Autodesk Inventor part; units mm, degrees
ref_plane "YZ Plane" through (0, 0, 0) normal (1, 0, 0) x (0, 1, 0)
ref_plane "XZ Plane" through (0, 0, 0) normal (0, 1, 0) x (-1, 0, 0)
ref_plane "XY Plane" through (0, 0, 0) normal (0, 0, 1) x (1, 0, 0)
sketch "Sketch1" plane through (0, 0, 0) normal (0, 0, 1) x (1, 0, 0)
  line L0 (-192.5, 35) -> (192.5, 35)
  line L1 (192.5, 35) -> (192.5, -55)
  line L2 (192.5, -55) -> (-192.5, -55)
  line L3 (-192.5, -55) -> (-192.5, 35)
  point P0 (0, 0)
  dimension "d0" = 385
  dimension "d1" = 192.5
  dimension "d2" = 90
  dimension "d3" = 55
extrude "Extrusion1" add sketch "Sketch1" along normal blind 7
sketch "Sketch2" plane through (0, 0, 0) normal (0, 0, -1) x (-1, 0, 0)
  line L0 (192.5, 35) -> (-192.5, 35)
  line L1 (-192.5, 35) -> (-192.5, -55)
  line L2 (-192.5, -55) -> (192.5, -55)
  line L3 (17.417, 16.6256) -> (17.417, -16.6484)
  line L4 (-192.5, 16.6256) -> (-192.5, -16.6484)
  line L5 (17.417, 35) -> (17.417, -55)
  line L6 (4.717, 16.6256) -> (4.717, -16.6484)
  line L7 (-171.164, 18.034) -> (-179.8, 18.034)
  line L8 (-179.8, 16.6256) -> (-179.8, -16.6484)
  line L9 (-179.8, 35) -> (-179.8, -55)
  line L10 (4.717, 35) -> (4.717, -55)
  point P0 (0, 0)
extrude "Extrusion2" add sketch "Sketch2" along normal blind 4.7408 contours L5 L3 L2 L10 L6 L0 | L9 L8 L2 L1 L0
sketch "Sketch3" plane through (0, 0, 0) normal (0, 0, -1) x (-1, 0, 0)
  line L0 (17.417, 35) -> (17.417, -55)
  line L1 (17.417, -55) -> (192.5, -55)
  line L2 (63.2414, 16.4628) -> (60.0979, -19.4679)
  line L3 (17.417, 35) -> (67.417, 35)
  line L4 (67.417, 35) -> (67.417, -55)
  line L5 (67.417, -55) -> (17.417, -55)
  line L6 (17.417, -55) -> (17.417, 35)
  line L7 (76.6696, -19.4) -> (76.6696, 30.6)
  line L8 (17.417, 35) -> (76.6696, 35)
  line L9 (76.6696, -55) -> (17.417, -55)
  line L10 (17.417, -55) -> (17.417, 35)
  circle A0 centre (83.6696, -4.5) radius 1.5
  circle A1 centre (83.6696, 10.5) radius 2
  line L11 (87.4689, -18.5) -> (87.4689, -24.5)
  line L12 (88.6696, -24.5) -> (87.4689, -24.5)
  line L13 (88.6696, 15.5) -> (88.6696, -24.5)
  line L14 (78.6696, 15.5) -> (88.6696, 15.5)
  line L15 (78.6696, -15.5) -> (78.6696, 15.5)
  line L16 (78.6696, -15.5) -> (84.4689, -15.5)
  arc A2 (87.4689, -18.5) -> (84.4689, -15.5) centre (84.4689, -18.5) ccw
  line L17 (67.417, 35) -> (78.6696, 35)
  line L18 (78.6696, 35) -> (78.6696, -55)
  line L19 (78.6696, -55) -> (67.417, -55)
  line L20 (67.417, -55) -> (67.417, 35)
  point P0 (0, 0)
  dimension "d8" = 50
  dimension "d11" = 0
extrude "Extrusion3" add sketch "Sketch3" along normal blind 7.3198 contours L3 L4 L1 L0 | L8 L17 L18 L15 L1 L4
sketch "Sketch6" plane through (-192.5, -55, 7) normal (-1, 0, 0) x (0, 0, 1)
  line L0 (-23, 0) -> (-23, 65)
  circle A0 centre (-28, 23.1) radius 1.2295
  circle A1 centre (-28, 53.1) radius 1.2295
  point P0 (-7, 55)
hole "Hole1" at (-192.5, -31.9, -21) at (-192.5, -1.9, -21) direction (1, 0, 0) diameter 3 end through all counterbore diameter 5.75 counterbore depth 3
sketch "Sketch8" plane through (0, 0, 7) normal (0, 0, 1) x (1, 0, 0)
  circle A0 centre (-57.2416, -1.1152) radius 2.0828
  circle A1 centre (-33.7068, 0.9439) radius 2.0828
  point P0 (0, 0)
hole "Hole3" [suppressed]
sketch "Sketch9" plane through (0, 0, -4.7408) normal (0, 0, -1) x (-1, 0, 0)
  circle A0 centre (11.067, -7.6314) radius 2.1844
  circle A1 centre (11.067, 7.6086) radius 2.1844
  circle A2 centre (-186.15, -7.6314) radius 2.1844
  circle A3 centre (-186.15, 7.6086) radius 2.1844
  point P0 (0, 0)
hole "Hole4" at (-11.067, -7.6314, -4.7408) at (-11.067, 7.6086, -4.7408) at (186.15, -7.6314, -4.7408) at (186.15, 7.6086, -4.7408) direction (0, 0, 1) diameter 3.302 depth 8 tip angle 118
sketch "Sketch10" plane through (0, 0, 0) normal (0, 0, -1) x (-1, 0, 0)
  line L0 (192.5, 35) -> (78.6696, 35)
  line L1 (178.6696, 15.5) -> (178.6696, -24.5)
  line L2 (178.6696, 35) -> (192.5, 35)
  line L3 (192.5, 35) -> (192.5, -55)
  line L4 (192.5, -55) -> (178.6696, -55)
  line L5 (178.6696, -55) -> (178.6696, 35)
  point P0 (0, 0)
extrude "Extrusion6" cut sketch "Sketch10" against normal blind 10
sketch "Sketch11" plane through (0, 0, 0) normal (0, 0, -1) x (-1, 0, 0)
  line L0 (178.6696, -55) -> (178.6696, 35)
  line L1 (178.6696, 35) -> (78.6696, 35)
  line L2 (78.6696, 35) -> (78.6696, -55)
  line L3 (78.6696, -55) -> (178.6696, -55)
  point P0 (0, 0)
extrude "Extrusion7" add sketch "Sketch11" along normal blind 7.3198
sketch "Sketch12" plane through (0, 0, -7.3198) normal (0, 0, -1) x (-1, 0, 0)
  circle A0 centre (173.6696, 10.5) radius 2
  line L0 (78.6696, 15.5) -> (178.6696, 15.5)
  line L1 (178.6696, 15.5) -> (178.6696, -24.5)
  line L2 (178.6696, -24.5) -> (78.6696, -24.5)
  line L3 (78.6696, -24.5) -> (78.6696, 15.5)
  circle A1 centre (173.6696, -44.5) radius 2.0242
  circle A2 centre (58.6696, 10.5) radius 2.0032
  circle A3 centre (58.6696, -44.5) radius 2.0032
  point P0 (0, 0)
  dimension "d126" = 55
  dimension "d127" = 115
hole "Hole5" at (-173.6696, 10.5, -7.3198) direction (0, 0, 1) diameter 2.459 depth 8.8 tip angle 118
sketch "Sketch13" plane through (0, 0, -7.3198) normal (0, 0, -1) x (-1, 0, 0)
  line L0 (171.6696, -6) -> (175.6696, -6)
  arc A0 (175.6696, -6) -> (175.6696, -3) centre (175.6696, -4.5) ccw
  line L1 (175.6696, -3) -> (171.6696, -3)
  arc A1 (171.6696, -3) -> (171.6696, -6) centre (171.6696, -4.5) ccw
  circle A2 centre (83.6696, -4.5) radius 1.5
  circle A3 centre (173.6696, 10.5) radius 2
  circle A4 centre (173.6696, -19.5) radius 2
  circle A5 centre (83.6696, 10.5) radius 2
  circle A6 centre (83.6696, -19.5) radius 2
  line L2 (78.6696, 15.5) -> (178.6696, 15.5)
  line L3 (178.6696, 15.5) -> (178.6696, -24.5)
  line L4 (178.6696, -24.5) -> (78.6696, -24.5)
  line L5 (78.6696, -24.5) -> (78.6696, 15.5)
  point P0 (0, 0)
  point P1 (173.6696, -4.5)
hole "Hole6" [suppressed]
sketch "Sketch14" plane through (0, 0, -7.3198) normal (0, 0, -1) x (-1, 0, 0)
  circle A0 centre (126.3, 25.4) radius 3.175
  circle A1 centre (151.7, 25.4) radius 3.175
  point P0 (0, 0)
  point P1 (100.9, 25.4)
  dimension "d63" = 50.8
hole "Hole7" at (-151.7, 25.4, -7.3198) at (-100.9, 25.4, -7.3198) direction (0, 0, 1) diameter 6.35 end through all counterbore diameter 9.652 counterbore depth 7
sketch "Sketch15" plane through (0, 0, -7.3198) normal (0, 0, -1) x (-1, 0, 0)
  line L0 (17.417, 35) -> (78.6696, 35)
  circle A0 centre (100.9, 25.4) radius 4.826
  point P0 (0, 0)
  point P1 (24.741, 27.9)
  point P2 (24.7, -22.9)
  dimension "d71" = 7.1
  dimension "d72" = 76.2
  dimension "d73" = 76.2
  dimension "d74" = 50.8
hole "Hole8" at (-24.741, 27.9, -7.3198) at (-24.7, -22.9, -7.3198) direction (0, 0, 1) diameter 6.35 end through all counterbore diameter 9.652 counterbore depth 7
sketch "Sketch17" plane through (0, 0, 0) normal (0, 0, -1) x (-1, 0, 0)
  line L0 (-179.8, -55) -> (4.717, -55)
  line L1 (4.717, 35) -> (-179.8, 35)
  line L2 (-109.583, 16.6256) -> (-109.583, -16.6484)
  line L3 (-96.883, 16.6256) -> (-96.883, -16.6484)
  line L4 (-96.883, 35) -> (-109.583, 35)
  line L5 (-109.583, 35) -> (-109.583, -55)
  line L6 (-109.583, -55) -> (-96.883, -55)
  line L7 (-96.883, -55) -> (-96.883, 35)
  point P0 (0, 0)
extrude "Extrusion8" add sketch "Sketch17" along normal blind 4.7408
sketch "Sketch18" plane through (0, 0, -4.7408) normal (0, 0, -1) x (-1, 0, 0)
  circle A0 centre (-103.233, -7.6314) radius 2.1844
  circle A1 centre (-103.233, 7.6086) radius 2.1844
  point P0 (0, 0)
hole "Hole10" at (103.233, -7.6314, -4.7408) at (103.233, 7.6086, -4.7408) direction (0, 0, 1) diameter 3.302 depth 8 tip angle 118
sketch "Sketch19" plane through (0, 0, -4.7408) normal (0, 0, -1) x (-1, 0, 0)
  line L0 (-192.5, -55) -> (-192.5, 35)
  line L1 (-179.8, -55) -> (-109.583, -55)
  line L2 (-109.583, 35) -> (-179.8, 35)
  line L3 (-109.583, 35) -> (-192.5, 35)
  line L4 (-192.5, 35) -> (-192.5, -55)
  line L5 (-192.5, -55) -> (-109.583, -55)
  line L6 (-109.583, -55) -> (-109.583, 35)
  point P0 (0, 0)
extrude "Extrusion9" cut sketch "Sketch19" against normal blind 25
sketch "Sketch20" plane through (0, 0, 0) normal (0, 0, -1) x (-1, 0, 0)
  circle A0 centre (24.7, -22.9) radius 4.826
  circle A1 centre (24.741, 27.9) radius 4.826
  point P0 (0, 0)
  point P1 (-76.9, -22.9)
  point P2 (-76.859, 27.9)
  dimension "d103" = 101.6
  dimension "d104" = 101.6
hole "Hole11" [suppressed]
hole "Hole12" [suppressed]
hole "Hole13" [suppressed]
hole "Hole14" at (-173.6696, -44.5, -7.3198) direction (0, 0, 1) diameter 2.459 depth 8.8 tip angle 118
hole "Hole15" at (-58.6696, 10.5, -7.3198) direction (0, 0, 1) diameter 2.459 depth 8.8 tip angle 118
hole "Hole16" at (-58.6696, -44.5, -7.3198) direction (0, 0, 1) diameter 2.459 depth 8.8 tip angle 118
properties part number "Oxxius laser subassy shortened baseplate"
Check sheet for the modelled part. Datum: model origin and axes. Units: mm. A direction names the side the tool comes from. Give positions to 0.01 mm unless a question says otherwise; leave off trailing zeros. Write each loop counter-clockwise with the first axis right and the second up, starting at its lowest first coordinate (ties: lowest second). Pieces come first, ordered by that corner, then holes. Notation, with made-up numbers: (21, -17.75) -> (51, -17.75) arc R18 ccw to (51, 6.25) -> close; hole circle Ø1 at (-6.5, 49). An arc over 180 degrees is marked (long way). One line per item, written item: value. Start each with the question number.
Item 1: Section check C-C on y = -34.5. Record the cut outline in (x, z), then the cut area to 3 significant figures.
Item 2: Material ranges on probe 1 along X at (y, z) = (-44.5, -1.25); probe 2 along X at (y, z) = (7.5, -3); probe 3 along Y at (x, z) = (-22.5, 6), recorded low to high. Write a range as from..to.
Item 3: Section check B-B on y = -22.9. Record the cut outline in (x, z) (3 decimals).
Item 4: Draft check along Y on faces 1 (the flat face through (-100, 29, -0.32)), 2 (the flat face through (-65, -55, 2)), 3 (the flat face through (-37, -9, 7)). Enter one of: +Y half, -Y half, draft (parallel to the pull), parting line (faces both ways), or undercut.
Item 5: Gauge pin test, flat ends, axial feed: pin 1 (2 mm diameter, centred on x = -11.07, y = 7.61, fed in from -Z); pin 2 (10 mm diameter, centred on x = -10.5, y = -12, fed in from -Z); pin 3 (5 mm diameter, centred on x = -151, y = 24, fed in from -Z). Record the tip position at first contact, or that the pin passes through.
Item 6: Section check D-D on x = 24. Record the cut outline in (y, z), then the cut area to 3 significant figures.
Item 7: Section check A-A on x = -151.7. Record the cut outline in (y, z) (3 decimals), then the cut area to 3 significant figures.
Item 8: Tool access check on faces 4 (the flat face through (-178.67, -11, 0)), 5 (the flat face through (109.583, -9, 1)), 6 (the cylindrical face through (-146.99, 24.35, -3.77)), 7 (the flat face through (-12.4, -9.4, -4.741)), 8 (the flat face through (-4.717, -9, -2)). Record the directions out of +Z, -Z, +X, -X, +Y, -Y that give a thin tool (end or side, any length) a straight path to the whole face; none if there is none.
Results list:
1. outline: (-178.67, -7.32) -> (-17.42, -7.32) -> (-17.42, -4.74) -> (-4.72, -4.74) -> (-4.72, 0) -> (96.88, 0) -> (96.88, -4.74) -> (109.58, -4.74) -> (109.58, 7) -> (-178.67, 7) -> close
1. area: 3,320 mm²
2. probe 1: -178.67..-174.9, -172.44..-59.9, -57.44..-4.72, 96.88..109.58
2. probe 2: -178.67..-12.71, -9.42..-4.72, 96.88..101.59, 104.88..109.58
2. probe 3: -55..-25.19, -20.61..25.65, 30.15..35
3. outline: (-178.67, -7.32) -> (-29.526, -7.32) -> (-29.526, -0.32) -> (-27.875, -0.32) -> (-27.875, 7) -> (-178.67, 7) -> close; (-21.525, -0.32) -> (-19.874, -0.32) -> (-19.874, -7.32) -> (-17.417, -7.32) -> (-17.417, -4.741) -> (-4.717, -4.741) -> (-4.717, 0) -> (96.883, 0) -> (96.883, -4.741) -> (109.583, -4.741) -> (109.583, 7) -> (-21.525, 7) -> close
4. face 1: undercut
4. face 2: -Y half
4. face 3: draft
5. pin 1: z = 3.65
5. pin 2: z = -4.74
5. pin 3: z = -0.32
6. outline: (-55, 0) -> (35, 0) -> (35, 7) -> (-55, 7) -> close
6. area: 630 mm²
7. outline: (-55, -7.32) -> (20.574, -7.32) -> (20.574, -0.32) -> (22.225, -0.32) -> (22.225, 7) -> (-55, 7) -> close; (28.575, -0.32) -> (30.226, -0.32) -> (30.226, -7.32) -> (35, -7.32) -> (35, 7) -> (28.575, 7) -> close
7. area: 1,170 mm²
8. face 4: +Z, -Z, -X, +Y, -Y
8. face 5: +Z, -Z, +X, +Y, -Y
8. face 6: -Z
8. face 7: -Z, +X, +Y, -Y
8. face 8: -Z, +Y, -Y
